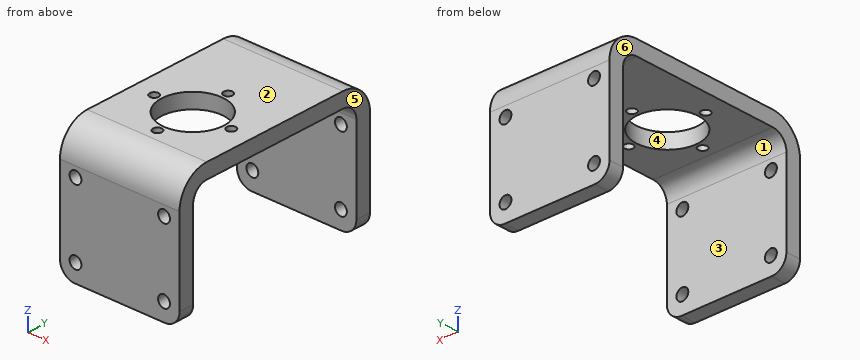
```python
from build123d import *

# Parameters (mm, degrees)
SKETCH1_W                = 40.35
SKETCH1_H                = 43.35
BOSS_EXTRUDE1_DEPTH      = 47
CUT_EXTRUDE2_DEPTH       = 102
FILLET1_R                = 10
CUT_EXTRUDE3_DEPTH       = 102
FILLET2_R                = 5
SKETCH7_R                = 10.5
SKETCH7_R_2              = 1.5
CUT_EXTRUDE5_DEPTH       = 10
SKETCH8_W                = 40.35
SKETCH8_H                = 43.175
BOSS_EXTRUDE2_DEPTH      = 38.35
BOSS_EXTRUDE2_DEPTH_BACK = 5
SKETCH6_R                = 2
CUT_EXTRUDE4_DEPTH       = 102
CUT_EXTRUDE4_DEPTH_BACK  = 102
CUT_EXTRUDE6_DEPTH       = 50
FILLET3_R                = 5
SKETCH10_R               = 10.5
SKETCH10_R_2             = 1.5
CUT_EXTRUDE7_DEPTH       = 50


with BuildPart() as part:
    # Sketch1 → Boss-Extrude1 (new body)
    with BuildSketch(Plane(origin=(0, 0, 0), x_dir=(1, 0, 0), z_dir=(0, 1, 0))):
        with Locations((-26.966212793, -29.108023223)):
            Rectangle(SKETCH1_W, SKETCH1_H)
    extrude(amount=BOSS_EXTRUDE1_DEPTH)

    # Sketch3 → Cut-Extrude2 (cut)
    with BuildSketch(Plane.XY.offset(50.783023223)):
        with BuildLine():
            Line((-47.141212793, 47), (-47.141212793, 26.825))
            ThreePointArc((-47.141212793, 26.825), (-41.232092103, 41.09087931), (-26.966212793, 47))
            Line((-26.966212793, 47), (-47.141212793, 47))
        make_face()
        with BuildLine():
            Line((-6.791212793, 47), (-26.966212793, 47))
            ThreePointArc((-26.966212793, 47), (-12.700333482, 41.09087931), (-6.791212793, 26.825))
            Line((-6.791212793, 26.825), (-6.791212793, 47))
        make_face()
    extrude(amount=-CUT_EXTRUDE2_DEPTH, mode=Mode.SUBTRACT)

    # Fillet1
    fillet1_edges = [part.edges().sort_by_distance(p)[0] for p in [
        (-26.966212793, 0, 50.783023223),
    ]]
    fillet(fillet1_edges, radius=FILLET1_R)

    # Sketch5 → Cut-Extrude3 (cut)
    with BuildSketch(Plane.ZY.offset(47.141212793)):
        with BuildLine():
            Line((-6.665763497, 5), (36.595559978, 5))
            Line((36.595559978, 5), (40.783023223, 5))
            ThreePointArc((40.783023223, 5), (44.318557129, 6.464466094), (45.783023223, 10))
            Line((45.783023223, 10), (45.783023223, 17.578484004))
            Line((45.783023223, 17.578484004), (45.783023223, 59.778436909))
            Line((45.783023223, 59.778436909), (-6.665763497, 59.778436909))
            Line((-6.665763497, 59.778436909), (-6.665763497, 5))
        make_face()
    extrude(amount=-CUT_EXTRUDE3_DEPTH, mode=Mode.SUBTRACT)

    # Fillet2
    fillet2_edges = [part.edges().sort_by_distance(p)[0] for p in [
        (-6.791212793, 2.5, 7.433023223),
        (-47.141212793, 2.5, 7.433023223),
    ]]
    fillet(fillet2_edges, radius=FILLET2_R)

    # Sketch7 → Cut-Extrude5 (cut)
    with BuildSketch(Plane.XY.offset(50.783023223)):
        with Locations((-26.966212793, 26.825)):
            Circle(SKETCH7_R)
        with Locations((-26.966212793, 39.825)):
            Circle(SKETCH7_R_2)
        with Locations((-13.966212793, 26.825)):
            Circle(SKETCH7_R_2)
        with Locations((-26.966212793, 13.825)):
            Circle(SKETCH7_R_2)
        with Locations((-39.966212793, 26.825)):
            Circle(SKETCH7_R_2)
    extrude(amount=-CUT_EXTRUDE5_DEPTH, mode=Mode.SUBTRACT)

    # Sketch8 → Boss-Extrude2 (add, two sides)
    with BuildSketch(Plane(origin=(0, 0, 45.783023223), x_dir=(-1, 0, 0), z_dir=(0, 0, -1))) as boss_extrude2_sk:
        with Locations((26.966212793, 48.4125)):
            Rectangle(SKETCH8_W, SKETCH8_H)
    extrude(amount=BOSS_EXTRUDE2_DEPTH)
    extrude(boss_extrude2_sk.sketch, amount=-BOSS_EXTRUDE2_DEPTH_BACK)

    # Sketch6 → Cut-Extrude4 (cut, two sides)
    with BuildSketch(Plane(origin=(0, 5, 0), x_dir=(1, 0, 0), z_dir=(0, 1, 0))) as cut_extrude4_sk:
        with Locations((-41.911212793, -13.433023223)):
            Circle(SKETCH6_R)
        with Locations((-12.021212793, -13.433023223)):
            Circle(SKETCH6_R)
        with Locations((-41.911212793, -37.493023223)):
            Circle(SKETCH6_R)
        with Locations((-12.021212793, -37.493023223)):
            Circle(SKETCH6_R)
    extrude(amount=CUT_EXTRUDE4_DEPTH, mode=Mode.SUBTRACT)
    extrude(cut_extrude4_sk.sketch, amount=-CUT_EXTRUDE4_DEPTH_BACK, mode=Mode.SUBTRACT)

    # Sketch9 → Cut-Extrude6 (cut)
    with BuildSketch(Plane(origin=(-6.791212793, 0, 0), x_dir=(0, 0, -1), z_dir=(1, 0, 0))):
        with BuildLine():
            Line((-7.433023223, 26.825), (-7.433023223, 65.000002288))
            Line((-7.433023223, 65.000002288), (-40.777808898, 65.000002288))
            ThreePointArc((-40.777808898, 65.000002288), (-44.31533911, 63.535699871), (-45.783023223, 59.99957135))
            Line((-45.783023223, 59.99957135), (-45.783023223, 26.825))
            Line((-45.783023223, 26.825), (-7.433023223, 26.825))
        make_face()
        with BuildLine():
            ThreePointArc((-50.783023223, 59.997178226), (-47.853264556, 67.070241334), (-40.780201449, 70))
            Line((-40.780201449, 70), (-50.783023223, 70))
            Line((-50.783023223, 70), (-50.783023223, 59.997178226))
        make_face()
    extrude(amount=-CUT_EXTRUDE6_DEPTH, mode=Mode.SUBTRACT)

    # Fillet3
    fillet3_edges = [part.edges().sort_by_distance(p)[0] for p in [
        (-47.141212793, 67.500001144, 7.433023223),
        (-6.791212793, 67.500001144, 7.433023223),
    ]]
    fillet(fillet3_edges, radius=FILLET3_R)

    # Sketch10 → Cut-Extrude7 (cut)
    with BuildSketch(Plane.XY.offset(50.783023223)):
        with Locations((-26.966212793, 26.825)):
            Circle(SKETCH10_R)
        with Locations((-13.966212793, 26.825)):
            Circle(SKETCH10_R_2)
        with Locations((-26.966212793, 13.825)):
            Circle(SKETCH10_R_2)
        with Locations((-39.966212793, 26.825)):
            Circle(SKETCH10_R_2)
        with Locations((-26.966212793, 39.825)):
            Circle(SKETCH10_R_2)
    extrude(amount=-CUT_EXTRUDE7_DEPTH, mode=Mode.SUBTRACT)


solid = part.part
```
CAD build for the part. Positions are in the model's coordinates, mm. Face numbers are marked on the shaded views. A direction names the side the tool comes from. Round coordinates to 2 decimals unless told otherwise and drop trailing zeros. Write each loop counter-clockwise with the first axis right and the second up, starting at its lowest first coordinate (ties: lowest second). Pieces come first, ordered by that corner, then holes. Notation, with made-up numbers: (41.25, 62) -> (75.25, 62) arc R22 cw to (75.25, 97) -> close; hole circle Ø5 at (48, 85). An arc over 180 degrees is marked (long way). Answer in a Markdown table with one row per item. Add a question column.
Item 1: Saw through at C-C, the plane x = -33.5. Write the cut outline in (y, z).
Item 2: Saw through at D-D, the plane y = 23. Write the cut outline in (x, z), then the cut area to 3 significant figures.
Item 3: Saw through at B-B, the plane z = 24. Write the cut outline in (x, y), then the cut area to 4 significant figures.
Item 4: Drill centre lines: line 1 (Y direction, x = -43, z = 15.5); line 2 (Y direction, x = -15.5, z = 44.5); line 3 (Z direction, x = -45.5, y = 30). Where is each one in solid material? Low to high. Write a range as from..to.
Item 5: Drop flat-ended pins along their axis: pin 1 Ø3 at (x, z) = (-41.91, 37.49) entering from -Y; pin 2 Ø3.5 at (x, y) = (-39.97, 26.82) entering from -Z. Give the stop position or say it passes through.
Item 6: Saw through at A-A, the plane x = -26.5. Write the cut outline in (y, z), then the cut area to 3 significant figures.
Item 7: Mould opens along X. For the marked faces 3, 4, 5 and 6 say: pulls with the +X half, pulls with the -X half, needs draft (parallel to the pull), parting line crosses it, or undercut.
Item 8: Which spindle directions (+Z, -Z, +X, -X, +Y, -Y) get a long thin tool onto all of the face, cutting with end or side? Do the marked faces 1 and 2. Say none if no direction does.
Findings below:
| question | item | result |
|---|---|---|
| 1 | outline | (0, 7.43) -> (5, 7.43) -> (5, 40.78) arc R5 cw to (10, 45.78) -> (18.61, 45.78) -> (18.61, 50.78) -> (10, 50.78) arc R10 ccw to (0, 40.78) -> close; (35.04, 45.78) -> (60, 45.78) arc R5.01 cw to (65, 40.78) -> (65, 7.43) -> (70, 7.43) -> (70, 40.78) arc R10 ccw to (60, 50.78) -> (35.04, 50.78) -> close |
| 2 | outline | (-47.14, 45.78) -> (-36.74, 45.78) -> (-36.74, 50.78) -> (-47.14, 50.78) -> close; (-17.19, 45.78) -> (-6.79, 45.78) -> (-6.79, 50.78) -> (-17.19, 50.78) -> close |
| 2 | area | 104 mm^2 |
| 3 | outline | (-47.14, 0) -> (-6.79, 0) -> (-6.79, 5) -> (-47.14, 5) -> close; (-47.14, 65) -> (-6.79, 65) -> (-6.79, 70) -> (-47.14, 70) -> close |
| 3 | area | 403.5 mm^2 |
| 4 | line 1 | y = 0..5, 65..70 |
| 4 | line 2 | y = 0.72..6.66, 63.34..69.28 |
| 4 | line 3 | z = 45.78..50.78 |
| 5 | pin 1 | passes through |
| 5 | pin 2 | stops at z = 45.78 |
| 6 | outline | (0, 7.43) -> (5, 7.43) -> (5, 40.78) arc R5 cw to (10, 45.78) -> (12.4, 45.78) -> (12.4, 50.78) -> (10, 50.78) arc R10 ccw to (0, 40.78) -> close; (15.25, 45.78) -> (16.34, 45.78) -> (16.34, 50.78) -> (15.25, 50.78) -> close; (37.31, 45.78) -> (38.4, 45.78) -> (38.4, 50.78) -> (37.31, 50.78) -> close; (41.25, 45.78) -> (60, 45.78) arc R5.01 cw to (65, 40.78) -> (65, 7.43) -> (70, 7.43) -> (70, 40.78) arc R10 ccw to (60, 50.78) -> (41.25, 50.78) -> close |
| 6 | area | 568 mm^2 |
| 7 | face 3 | needs draft |
| 7 | face 4 | undercut |
| 7 | face 5 | pulls with the +X half |
| 7 | face 6 | pulls with the -X half |
| 8 | face 1 | -Z, +X, -X |
| 8 | face 2 | +Z, +X, -X, +Y, -Y |
